```python
from build123d import *

# Parameters (mm, degrees)
F0_W     = 25.4
F0_H     = 19.05
F1_DEPTH = 19.05
F3_DEPTH = 19.051


with BuildPart() as f1:
    # F0 (on Front) → F1 (new body)
    with BuildSketch(Plane.XZ):
        Polygon((93.3704, -10.24128), (-17.78, 189.60592), (-84.4804, 189.60592), (-84.4804, -184.48528), (-59.0804, -184.48528), (-33.6804, -184.48528), (42.5704, -184.48528), (67.9704, -184.48528), (93.3704, -184.48528), align=None)
        with Locations((55.2704, -194.01028)):
            Rectangle(F0_W, F0_H)
        with Locations((-46.3804, -194.01028)):
            Rectangle(F0_W, F0_H)
    extrude(amount=F1_DEPTH)

    # F2 (on face) → F3 (cut, through all)
    with BuildSketch(Plane.XZ.offset(19.05)):
        Polygon((-24.446551, 97.077993), (-49.138289, 141.473467), (-65.786592, 132.214065), (-41.094854, 87.818592), align=None)
        Polygon((49.628662, -36.108428), (32.98036, -45.367829), (57.672097, -89.763303), (74.3204, -80.503901), align=None)
    extrude(amount=-F3_DEPTH, mode=Mode.SUBTRACT)


solid = f1.part
```
The listing builds one solid part. Answer for the finished solid, in the listing's coordinates (mm). A direction names the side the tool comes from. Give positions to 0.01 mm unless a question says otherwise; leave off trailing zeros. Loops run counter-clockwise (first coordinate to the right, second up) from the corner with the lowest first, then second, coordinate; pieces in that order, holes last. Notation, with made-up numbers: (-40, 60.5) - (10, 60.5) arc R29 cw to (10, 85.5) - close; hole circle Ø2 at (85, 56.5). An arc over 180 degrees is marked (long way). Return JSON: item names as keys, results as strings. Group by question number.
1. Find section A-A (x = 53.5). Write down the section's boundary in (y, z).
2. Find section D-D (x = -73.5). Write down the section's boundary in (y, z), then the cut area to 3 significant figures.
3. Given pin 1 Ø5.5 at (y, z) = (-6, -198) entering from +X; pin 2 Ø9.5 at (y, z) = (-9, -196.5) entering from -X; pin 3 Ø5.5 at (x, y) = (-12, -13.5) entering from -Z, each flat-ended and moving along its own axis, determine where each tip first touches the part or whether it passes through.
4. Which of the six approach directions +Z, -Z, +X, -X, +Y, -Y give full straight-line access (tool end or side, diameter ignored) to faces 1 (the flat face through (-59.08, -9, -194)), 2 (the flat face through (67.97, -9, -194)), 3 (the flat face through (65.88, -9.66, -85.2))?
5. Straight lines are drawn through the part: line 1 (Z direction, x = -32, y = -15); line 2 (Z direction, x = -72.5, y = -10); line 3 (X direction, y = -7.5, z = 106). For each, find the intervals that lie inside material, in ascending order. Write a range as [from, to].
6. Find section C-C (z = 114). Write down the section's boundary in (x, y).
7. Find section B-B (y = -3). Write down the section's boundary in (x, z), then the cut area to 3 significant figures.
8. Determine the mould class of faces 4 (the flat face through (-53.6, -9.7, 110.3)), 5 (the flat face through (80, -9, -184.485)), 6 (the flat face through (42.57, -9, -194)), 7 (the flat face through (45.15, -9.66, -67.25)) for opening direction Z: pulls with the +Z half, pulls with the -Z half, needs draft (parallel to the pull), parting line crosses it, or undercut.
Verdict:
{
 "1": {"outline": "(-19.05, -203.54) - (0, -203.54) - (0, -82.26) - (-19.05, -82.26) - close; (-19.05, -43.07) - (0, -43.07) - (0, 61.45) - (-19.05, 61.45) - close"},
 "2": {"outline": "(-19.05, -184.49) - (0, -184.49) - (0, 189.61) - (-19.05, 189.61) - close", "area": "7,130 mm^2"},
 "3": {"pin 1": "stops at x = 67.97", "pin 2": "stops at x = -59.08", "pin 3": "stops at z = -184.49"},
 "4": {"face 1": "-Z, -X, +Y, -Y", "face 2": "-Z, +X, +Y, -Y", "face 3": "+Y, -Y"},
 "5": {"line 1": "z = [-184.49, 92.88], [110.66, 189.61]", "line 2": "z = [-184.49, 189.61]", "line 3": "x = [-84.48, -51.21], [-29.41, 28.72]"},
 "6": {"outline": "(-84.48, -19.05) - (-55.66, -19.05) - (-55.66, 0) - (-84.48, 0) - close; (-33.86, -19.05) - (24.27, -19.05) - (24.27, 0) - (-33.86, 0) - close"},
 "7": {"outline": "(-84.48, -184.49) - (-59.08, -184.49) - (-59.08, -203.54) - (-33.68, -203.54) - (-33.68, -184.49) - (42.57, -184.49) - (42.57, -203.54) - (67.97, -203.54) - (67.97, -184.49) - (93.37, -184.49) - (93.37, -10.24) - (-17.78, 189.61) - (-84.48, 189.61) - close; hole (-65.79, 132.21) - (-41.09, 87.82) - (-24.45, 97.08) - (-49.14, 141.47) - close; hole (32.98, -45.37) - (57.67, -89.76) - (74.32, -80.5) - (49.63, -36.11) - close", "area": "54,500 mm^2"},
 "8": {"face 4": "undercut", "face 5": "pulls with the -Z half", "face 6": "needs draft", "face 7": "undercut"}
}
